Drawing for the job (mm, zero at the part's lowest x, y, z). Give positions to 0.01 mm unless a question says otherwise; leave off trailing zeros. Write each loop counter-clockwise with the first axis right and the second up, starting at its lowest first coordinate (ties: lowest second). Pieces come first, ordered by that corner, then holes. Notation, with made-up numbers: M 46.5,56.25 L 90.5,56.25 A13 cw 90.5,73.25 Z; hole C 42.5,-5 d1. An arc over 180 degrees is marked long. Use CSV: the item, a comma, the result in double quotes. Start each with the question number.
1. Drill centre lines: line 1 along Y through (x, z) = (25, 11); line 2 along Y through (x, z) = (45, 6); line 3 along Z through (x, y) = (28.5, 55.5). Where is each one in solid material? Low to high. Write a range as from..to.
2. Drop flat-ended pins along their axis: pin 1 Ø1.5 at (x, y) = (5, 57.05) entering from +Z; pin 2 Ø5 at (x, y) = (22.5, 3.5) entering from +Z; pin 3 Ø12 at (x, y) = (28, 19) entering from +Z. Give the stop position or say it passes through.
3. Band-saw the part on C-C, the plane x = 25. List the corners of the cut face in (y, z).
4. Band-saw the part on A-A, the plane x = 5. List the corners of the cut face in (y, z), then the cut area to 4 significant figures.
5. Band-saw the part on B-B, the plane y = 2.95. List the corners of the cut face in (x, z).
6. Band-saw the part on D-D, the plane y = 30. List the corners of the cut face in (x, z), then the cut area to 3 significant figures.
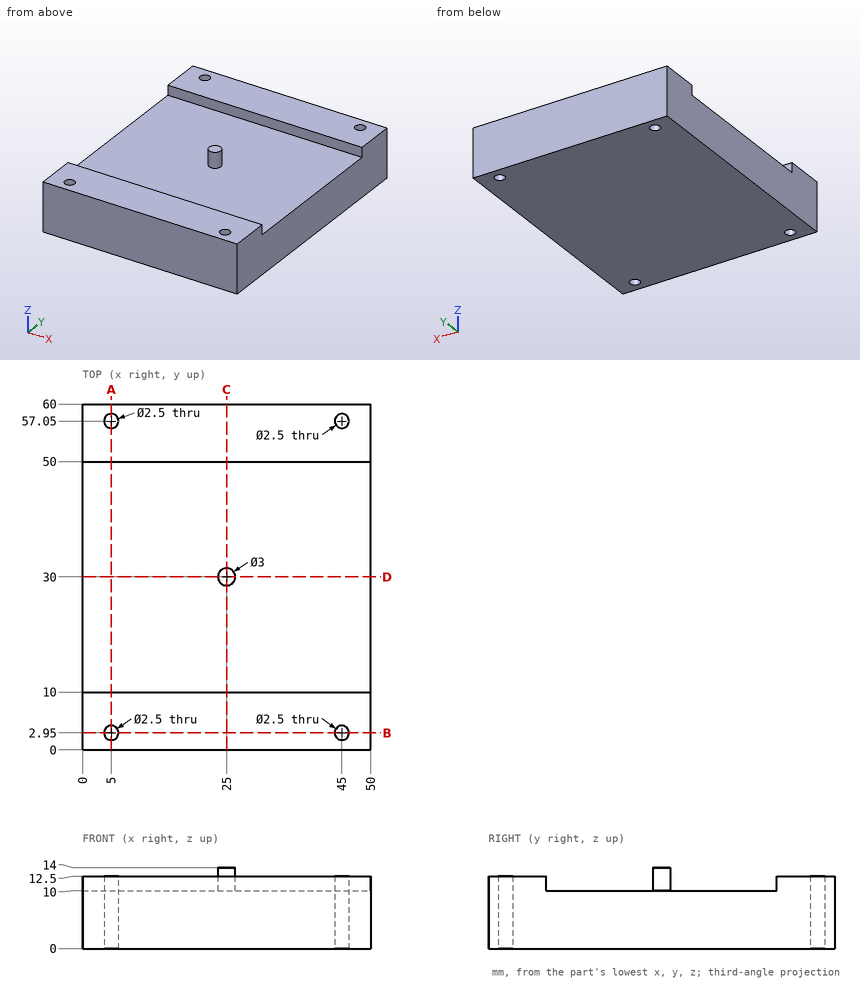
Output:
1,line 1,"y = 0..10, 28.5..31.5, 50..60"
1,line 2,"y = 0..1.7, 4.2..55.8, 58.3..60"
1,line 3,"z = 0..12.5"
2,pin 1,"passes through"
2,pin 2,"stops at z = 12.5"
2,pin 3,"stops at z = 10"
3,outline,"M 0,0 L 60,0 L 60,12.5 L 50,12.5 L 50,10 L 31.5,10 L 31.5,14 L 28.5,14 L 28.5,10 L 10,10 L 10,12.5 L 0,12.5 Z"
4,outline,"M 0,0 L 1.7,0 L 1.7,12.5 L 0,12.5 Z; M 4.2,0 L 55.8,0 L 55.8,12.5 L 50,12.5 L 50,10 L 10,10 L 10,12.5 L 4.2,12.5 Z; M 58.3,0 L 60,0 L 60,12.5 L 58.3,12.5 Z"
4,area,"587.5 mm²"
5,outline,"M 0,0 L 3.75,0 L 3.75,12.5 L 0,12.5 Z; M 6.25,0 L 43.75,0 L 43.75,12.5 L 6.25,12.5 Z; M 46.25,0 L 50,0 L 50,12.5 L 46.25,12.5 Z"
6,outline,"M 0,0 L 50,0 L 50,10 L 26.5,10 L 26.5,14 L 23.5,14 L 23.5,10 L 0,10 Z"
6,area,"512 mm²"
